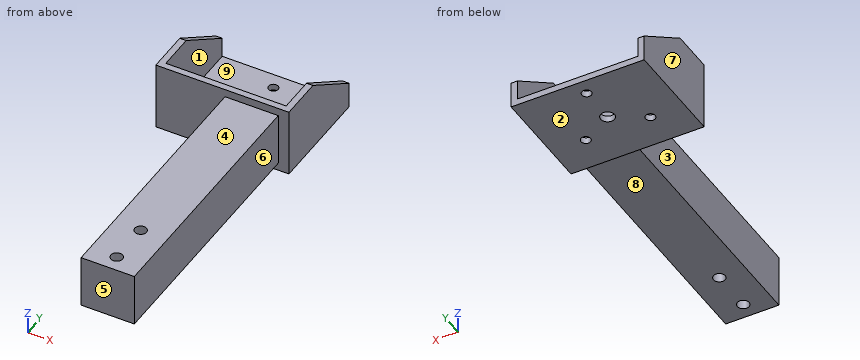
from build123d import *

# Parameters (mm, degrees)
SKETCH_1_W               = 125
SKETCH_1_H               = 100
EXTRUDE_1_DEPTH          = 65
SHELL_1_T                = -6
CUT_EXTRUDE_1_REACH      = 174.772
SKETCH_3_W               = 50
SKETCH_3_H               = 50
EXTRUDE_2_DEPTH          = 240
SKETCH_4_R               = 5.5
CUT_EXTRUDE_2_DEPTH      = 240
SKETCH_5_R               = 6.5
CUT_EXTRUDE_5_DEPTH      = 240
SKETCH_6_R               = 4.5
CUT_EXTRUDE_6_DEPTH      = 240
PATTERN_CIRCULAR_1_COUNT = 3


with BuildPart() as part:
    # 草图1 → 凸台-拉伸1 (new body)
    with BuildSketch(Plane.XY):
        with Locations((62.5, 50)):
            Rectangle(SKETCH_1_W, SKETCH_1_H)
    extrude(amount=EXTRUDE_1_DEPTH)

    # 抽壳1
    shell_1_openings = [part.faces().sort_by_distance(p)[0] for p in [
        (62.5, 50, 65),
        (62.5, 100, 32.5),
    ]]
    offset(amount=SHELL_1_T, openings=shell_1_openings, kind=Kind.INTERSECTION)

    # 切除-拉伸1: up to this face of the body (flat: up to its plane)
    cut_extrude_1_end = Plane(part.part.faces().sort_by_distance((0, 50, 32.5))[0])
    # 草图2 → 切除-拉伸1 (cut, up to the picked face)
    with BuildSketch(Plane(origin=(125, 0, 0), x_dir=(0, 0, -1), z_dir=(1, 0, 0)), mode=Mode.PRIVATE) as cut_extrude_1_sk1:
        Polygon((-65, 100), (-25, 100), (-65, 40), align=None)
    cut_extrude_1_tool1 = split(extrude(cut_extrude_1_sk1.sketch, amount=-CUT_EXTRUDE_1_REACH, mode=Mode.PRIVATE), bisect_by=cut_extrude_1_end, keep=Keep.BOTH, mode=Mode.PRIVATE)
    add(cut_extrude_1_tool1.solids().sort_by(Axis((125, 80, 51.666667), (-1, 0, 0)))[0], mode=Mode.SUBTRACT)

    # 草图3 → 凸台-拉伸2 (add)
    with BuildSketch(Plane.XZ):
        with Locations((90, 32.5)):
            Rectangle(SKETCH_3_W, SKETCH_3_H)
    extrude(amount=EXTRUDE_2_DEPTH)

    # 草图4 → 切除-拉伸2 (cut)
    with BuildSketch(Plane.XY.offset(57.5)):
        with Locations((90, -225)):
            Circle(SKETCH_4_R)
        with Locations((90, -185)):
            Circle(SKETCH_4_R)
    extrude(amount=-CUT_EXTRUDE_2_DEPTH, mode=Mode.SUBTRACT)

    # 草图5 → 切除-拉伸5 (cut)
    with BuildSketch(Plane(origin=(0, 0, 0), x_dir=(-1, 0, 0), z_dir=(0, 0, -1))):
        with Locations((-62.5, 50)):
            Circle(SKETCH_5_R)
    extrude(amount=-CUT_EXTRUDE_5_DEPTH, mode=Mode.SUBTRACT)

    # 草图6 → 切除-拉伸6 (cut)
    with BuildSketch(Plane(origin=(0, 0, 0), x_dir=(-1, 0, 0), z_dir=(0, 0, -1))):
        with Locations((-62.5, 85)):
            Circle(SKETCH_6_R)
    cut_extrude_6 = extrude(amount=-CUT_EXTRUDE_6_DEPTH, mode=Mode.SUBTRACT)

    # 阵列(圆周)1: 切除-拉伸6 ×3 about axis
    pattern_circular_1_axis = Axis((62.5, 50, 0), (0, 0, 1))
    for i in range(1, PATTERN_CIRCULAR_1_COUNT):
        add(cut_extrude_6.rotate(pattern_circular_1_axis, i * 360 / PATTERN_CIRCULAR_1_COUNT), mode=Mode.SUBTRACT)


solid = part.part
Could you check a few things on this model? Use its own coordinates, in mm. Face numbers are marked on the shaded views. A direction names the side the tool comes from. Give positions to 0.01 mm unless a question says otherwise; leave off trailing zeros. Order: outer loops, then holes, each group sorted by start corner. A loop starts at its lowest first (then second) coordinate and runs counter-clockwise, first axis right, second up. Notation, with made-up numbers: (30, -3.5) - (75, -3.5) arc R26 ccw to (75, 35.5) - close; hole circle Ø4 at (9.25, 23.25). An arc over 180 degrees is marked (long way). One line per question, with ' | ' between items. Start each with the question number.
Item 1: I want a section at B-B on z = 13. Write out the boundary of the cut face in (x, y).
Item 2: I want a section at A-A on y = 32.5. Write out the boundary of the cut face in (x, z).
Item 3: For the marked faces 1, 2, 3, 4 and 5, which set-ups out of +Z, -Z, +X, -X, +Y, -Y let a thin tool reach every point of the face, with its end or its side?
Item 4: I'm going to push flat-ended pins straight in: pin 1 Ø17.5 at (x, y) = (90, -225) entering from +Z; pin 2 Ø6 at (x, y) = (84.5, 47.5) entering from +Z; pin 3 Ø15 at (x, y) = (84, -63) entering from -Z; pin 4 Ø7 at (x, y) = (32.19, 32.5) entering from -Z. Where does each tip first touch, or does it pass through?
Item 5: I need wall thicknesses on probe 1 along X at (y, z) = (32, 4); probe 2 along Y at (x, z) = (62, 1); probe 3 along Y at (x, z) = (90, 41.5). Which ranges of each line are inside material? Lowest first, please. Write a range as [from, to].
Item 6: Thinking about a two-plate mould opening in X: for the marked faces 6, 7, 8 and 9, which applies, pulls with the +X half, pulls with the -X half, needs draft (parallel to the pull), parting line crosses it, or undercut?
Item 7: I want a section at D-D on x = 105. Write out the boundary of the cut face in (y, z).
Item 8: I want a section at C-C on y = 85. Write out the boundary of the cut face in (x, z), then the cut area to 3 significant figures.
Verdict:
1) outline: (0, 0) - (65, 0) - (65, -240) - (115, -240) - (115, 0) - (125, 0) - (125, 100) - (119, 100) - (119, 6) - (6, 6) - (6, 100) - (0, 100) - close; hole circle Ø11 at (90, -225); hole circle Ø11 at (90, -185)
2) outline: (0, 0) - (27.69, 0) - (27.69, 6) - (6, 6) - (6, 65) - (0, 65) - close; (36.69, 0) - (88.31, 0) - (88.31, 6) - (36.69, 6) - close; (97.31, 0) - (125, 0) - (125, 65) - (119, 65) - (119, 6) - (97.31, 6) - close
3) face 1: +Z, +Y | face 2: -Z, +X, -X, +Y, -Y | face 3: +Z, -Z, -X, -Y | face 4: +Z, +X, -X, -Y | face 5: +Z, -Z, +X, -X, -Y
4) pin 1: z = 57.5 | pin 2: z = 6 | pin 3: z = 7.5 | pin 4: through
5) probe 1: [0, 27.72], [36.66, 88.34], [97.28, 125] | probe 2: [0, 43.52], [56.48, 80.53], [89.47, 100] | probe 3: [-240, -230.5], [-219.5, -190.5], [-179.5, 6]
6) face 6: pulls with the +X half | face 7: pulls with the -X half | face 8: needs draft | face 9: undercut
7) outline: (-240, 7.5) - (0, 7.5) - (0, 0) - (100, 0) - (100, 6) - (6, 6) - (6, 65) - (0, 65) - (0, 57.5) - (-240, 57.5) - close
8) outline: (0, 0) - (58, 0) - (58, 6) - (6, 6) - (6, 35) - (0, 35) - close; (67, 0) - (125, 0) - (125, 35) - (119, 35) - (119, 6) - (67, 6) - close | area: 1,040 mm^2
